```python
from build123d import *

# Parameters (mm, degrees)
SKETCH_1_W          = 90
SKETCH_1_H          = 55
EXTRUDE_1_DEPTH     = 2
SKETCH_2_R          = 1.55
CUT_EXTRUDE_1_DEPTH = 2
SKETCH_3_R          = 1.55
CUT_EXTRUDE_2_DEPTH = 10
SKETCH_4_R          = 2.05
CUT_EXTRUDE_3_DEPTH = 10
SKETCH_5_R          = 1.55
CUT_EXTRUDE_4_DEPTH = 10
SKETCH_6_W          = 7
SKETCH_6_H          = 20
CUT_EXTRUDE_5_DEPTH = 10
SKETCH_7_W          = 12
SKETCH_7_H          = 15
CUT_EXTRUDE_6_DEPTH = 10
SKETCH_8_W          = 7
SKETCH_8_H          = 8
SKETCH_8_W_2        = 12
SKETCH_8_H_2        = 10
CUT_EXTRUDE_7_DEPTH = 10
FILLET_1_R          = 1


with BuildPart() as part:
    # 草图1 → 凸台-拉伸1 (new body)
    with BuildSketch(Plane(origin=(0, 0, 0), x_dir=(1, 0, 0), z_dir=(0, 1, 0))):
        Rectangle(SKETCH_1_W, SKETCH_1_H)
    extrude(amount=EXTRUDE_1_DEPTH)

    # 草图2 → 切除-拉伸1 (cut)
    with BuildSketch(Plane(origin=(0, 2, 0), x_dir=(1, 0, 0), z_dir=(0, 1, 0))):
        with Locations(Location((0, -12, 0), (0, 0, 270))):
            Circle(SKETCH_2_R)
        with Locations(Location((0, 12, 0), (0, 0, 90))):
            Circle(SKETCH_2_R)
        with Locations(Location((0, 0, 0), (0, 0, 270))):
            Circle(SKETCH_2_R)
        with Locations(Location((42, 12, 0), (0, 0, 270))):
            Circle(SKETCH_2_R)
        with Locations(Location((42, 0, 0), (0, 0, 270))):
            Circle(SKETCH_2_R)
        with Locations(Location((42, -12, 0), (0, 0, 90))):
            Circle(SKETCH_2_R)
    extrude(amount=-CUT_EXTRUDE_1_DEPTH, mode=Mode.SUBTRACT)

    # 草图3 → 切除-拉伸2 (cut)
    with BuildSketch(Plane(origin=(0, 2, 0), x_dir=(1, 0, 0), z_dir=(0, 1, 0))):
        with Locations(Location((35, 21, 0), (0, 0, 270))):
            Circle(SKETCH_3_R)
        with Locations(Location((35, -21, 0), (0, 0, 270))):
            Circle(SKETCH_3_R)
    extrude(amount=-CUT_EXTRUDE_2_DEPTH, mode=Mode.SUBTRACT)

    # 草图4 → 切除-拉伸3 (cut)
    with BuildSketch(Plane(origin=(0, 2, 0), x_dir=(1, 0, 0), z_dir=(0, 1, 0))):
        with Locations(Location((-32, 21, 0), (0, 0, 270))):
            Circle(SKETCH_4_R)
        with Locations(Location((-32, -21, 0), (0, 0, 270))):
            Circle(SKETCH_4_R)
        with Locations(Location((10, 21, 0), (0, 0, 270))):
            Circle(SKETCH_4_R)
        with Locations(Location((10, -21, 0), (0, 0, 270))):
            Circle(SKETCH_4_R)
    extrude(amount=-CUT_EXTRUDE_3_DEPTH, mode=Mode.SUBTRACT)

    # 草图5 → 切除-拉伸4 (cut)
    with BuildSketch(Plane(origin=(0, 2, 0), x_dir=(1, 0, 0), z_dir=(0, 1, 0))):
        with Locations(Location((-42, 9, 0), (0, 0, 270))):
            Circle(SKETCH_5_R)
        with Locations(Location((-42, -9, 0), (0, 0, 270))):
            Circle(SKETCH_5_R)
        with Locations(Location((-22, -9, 0), (0, 0, 270))):
            Circle(SKETCH_5_R)
        with Locations(Location((-22, 9, 0), (0, 0, 270))):
            Circle(SKETCH_5_R)
    extrude(amount=-CUT_EXTRUDE_4_DEPTH, mode=Mode.SUBTRACT)

    # 草图6 → 切除-拉伸5 (cut)
    with BuildSketch(Plane(origin=(0, 2, 0), x_dir=(1, 0, 0), z_dir=(0, 1, 0))):
        with Locations((31, 0)):
            Rectangle(SKETCH_6_W, SKETCH_6_H)
    extrude(amount=-CUT_EXTRUDE_5_DEPTH, mode=Mode.SUBTRACT)

    # 草图7 → 切除-拉伸6 (cut)
    with BuildSketch(Plane(origin=(0, 2, 0), x_dir=(1, 0, 0), z_dir=(0, 1, 0))):
        with Locations((-11, 0)):
            Rectangle(SKETCH_7_W, SKETCH_7_H)
    extrude(amount=-CUT_EXTRUDE_6_DEPTH, mode=Mode.SUBTRACT)

    # 草图8 → 切除-拉伸7 (cut)
    with BuildSketch(Plane(origin=(0, 2, 0), x_dir=(1, 0, 0), z_dir=(0, 1, 0))):
        with Locations((-20.5, 0)):
            Rectangle(SKETCH_8_W, SKETCH_8_H)
        with Locations((10, 0)):
            Rectangle(SKETCH_8_W_2, SKETCH_8_H_2)
    extrude(amount=-CUT_EXTRUDE_7_DEPTH, mode=Mode.SUBTRACT)

    # 圆角1
    fillet_1_edges = [part.edges().sort_by_distance(p)[0] for p in [
        (27.5, 1, 10),
        (27.5, 1, -10),
        (34.5, 1, -10),
        (34.5, 1, 10),
        (-5, 1, -7.5),
        (-5, 1, 7.5),
        (-17, 1, 7.5),
        (-17, 1, -7.5),
        (-17, 1, -4),
        (-17, 1, 4),
        (-24, 1, 4),
        (-24, 1, -4),
        (16, 1, -5),
        (16, 1, 5),
        (4, 1, 5),
        (4, 1, -5),
    ]]
    fillet(fillet_1_edges, radius=FILLET_1_R)


solid = part.part
```
The model under review builds one solid part; all positions refer to its coordinate system, in mm. A direction names the side the tool comes from. Give positions to 0.01 mm unless a question says otherwise; leave off trailing zeros. Write each loop counter-clockwise with the first axis right and the second up, starting at its lowest first coordinate (ties: lowest second). Pieces come first, ordered by that corner, then holes. Notation, with made-up numbers: M 24.25,-31.75 L 42.25,-31.75 A25 ccw 42.25,0.25 Z; hole C 60,64 d10. An arc over 180 degrees is marked long. Write each question's results on one line, items separated by ' | '. Start each with the question number.
1. We need section D-D (y = 1.35). Count the separate pieces of the cut face and the enclosed holes in it, and give its area (3 significant figures).
2. We need section B-B (x = -22). Write out the cut boundary in (y, z), and give its area (3 significant figures).
3. We need section C-C (x = -32). Write out the cut boundary in (y, z).
4. For faces 1 (the flat face through (27.5, 1, 0)), 2 (the flat face through (-1, 2, -6)), list the 3-axis set-ups (+Z, -Z, +X, -X, +Y, -Y) from which the entire face can be reached by the end or side of a thin tool; tool diameter is ignored.
5. Mouldability with a two-part tool opening along Z and no side actions: class faces 3 (the flat face through (-1, 1, 27.5)), 4 (the flat face through (-1, 0, -6)), 5 (the cylindrical face through (-20.463, 1.014, -9.202)) as released by +Z, released by -Z, zero draft, split by the parting line, or undercut.
6. Insertion check: pin 1 Ø5.5 at (x, z) = (-32, -21) entering from +Y. The pin has a flat end and moves straight along its axis. Give the tip position at first contact, or say it passes through.
7. We need section A-A (z = -21). Write out the cut boundary in (x, y).
8. For probe 1 along X at (y, z) = (1.75, -21); probe 2 along X at (y, z) = (1.3, 0); probe 3 along X at (y, z) = (0.45, -9), list the stretches that pass through material, from the lowest coordinate up. Write a range as [from, to].
Results found:
1) separate pieces: 1 | enclosed holes: 19 | area: 4,310 mm^2
2) outline: M 0,-27.5 L 2,-27.5 L 2,-10.55 L 0,-10.55 Z; M 0,-7.45 L 2,-7.45 L 2,-4 L 0,-4 Z; M 0,4 L 2,4 L 2,7.45 L 0,7.45 Z; M 0,10.55 L 2,10.55 L 2,27.5 L 0,27.5 Z | area: 81.6 mm^2
3) outline: M 0,-27.5 L 2,-27.5 L 2,-23.05 L 0,-23.05 Z; M 0,-18.95 L 2,-18.95 L 2,18.95 L 0,18.95 Z; M 0,23.05 L 2,23.05 L 2,27.5 L 0,27.5 Z
4) face 1: +Y, -Y | face 2: +Z, -Z, +X, -X, +Y
5) face 3: released by +Z | face 4: zero draft | face 5: undercut
6) pin 1: stops at y = 2
7) outline: M -45,0 L -34.05,0 L -34.05,2 L -45,2 Z; M -29.95,0 L 7.95,0 L 7.95,2 L -29.95,2 Z; M 12.05,0 L 33.45,0 L 33.45,2 L 12.05,2 Z; M 36.55,0 L 45,0 L 45,2 L 36.55,2 Z
8) probe 1: x = [-45, -34.05], [-29.95, 7.95], [12.05, 33.45], [36.55, 45] | probe 2: x = [-45, -24], [-5, -1.55], [1.55, 4], [16, 27.5], [34.5, 40.45], [43.55, 45] | probe 3: x = [-45, -43.55], [-40.45, -23.55], [-20.45, 27.5], [34.5, 45]
